```python
from build123d import *

# Parameters (mm, degrees)
F0_R     = 57.15
F0_R_2   = 5
F1_DEPTH = 15
F2_R     = 9.345244
F2_R_2   = 5.10775
F3_DEPTH = 15
F4_R     = 3
F5_DEPTH = 12.7
F6_R     = 1.5
F7_DEPTH = 10


with BuildPart() as f1:
    # F0 (on Front) → F1 (new body)
    with BuildSketch(Plane.XZ):
        Circle(F0_R)
        Circle(F0_R_2, mode=Mode.SUBTRACT)
    extrude(amount=F1_DEPTH)

    # F2 (on face) → F3 (join)
    with BuildSketch(Plane.XZ.offset(15)):
        Circle(F2_R)
        Circle(F2_R_2, mode=Mode.SUBTRACT)
    extrude(amount=F3_DEPTH)

    # F4 (on Top) → F5 (cut, symmetric)
    with BuildSketch(Plane.XY):
        with Locations((0, -23.08)):
            Circle(F4_R)
    extrude(amount=F5_DEPTH, both=True, mode=Mode.SUBTRACT)

    # F6 (on face) → F7 (join)
    with BuildSketch(Plane(origin=(0, 0, 0), x_dir=(-1, 0, 0), z_dir=(0, 1, 0))):
        with Locations((0, 10)):
            Circle(F6_R)
        with Locations((7.071068, 7.071068)):
            Circle(F6_R)
        with Locations((10, 0)):
            Circle(F6_R)
        with Locations((7.071068, -7.071068)):
            Circle(F6_R)
        with Locations((0, -10)):
            Circle(F6_R)
        with Locations((-10, 0)):
            Circle(F6_R)
        with Locations((-7.071068, -7.071068)):
            Circle(F6_R)
        with Locations((-7.071068, 7.071068)):
            Circle(F6_R)
    extrude(amount=F7_DEPTH)


solid = f1.part
```
Source: CAD feature listing. Evaluate the final solid. Frame: model axes, mm. A direction names the side the tool comes from. Round coordinates to 2 decimals unless told otherwise and drop trailing zeros. Loops run counter-clockwise (first coordinate to the right, second up) from the corner with the lowest first, then second, coordinate; pieces in that order, holes last. Notation, with made-up numbers: (-0.5, 33.5) - (40.5, 33.5) arc R19 ccw to (40.5, 44.5) - close; hole circle Ø4 at (-24, 56). An arc over 180 degrees is marked (long way). Use CSV: the item, a comma, the result in double quotes.
Q1. Section query C-C, the plane y = 3. Output: boundary loops of the cut face in (x, z).
Reported:
outline,"circle Ø3 at (-10, 0); circle Ø3 at (-7.07, -7.07); circle Ø3 at (-7.07, 7.07); circle Ø3 at (0, -10); circle Ø3 at (0, 10); circle Ø3 at (7.07, -7.07); circle Ø3 at (7.07, 7.07); circle Ø3 at (10, 0)"
Q2. Section query A-A, the plane z = 0. Output: boundary loops of the cut face in (x, y).
Reported:
outline,"(-57.15, -15) - (-9.35, -15) - (-9.35, -30) - (-5.11, -30) - (-5.11, -15) - (-5, -15) - (-5, 0) - (-8.5, 0) - (-8.5, 10) - (-11.5, 10) - (-11.5, 0) - (-57.15, 0) - close; (5, -15) - (5.11, -15) - (5.11, -30) - (9.35, -30) - (9.35, -15) - (57.15, -15) - (57.15, 0) - (11.5, 0) - (11.5, 10) - (8.5, 10) - (8.5, 0) - (5, 0) - close"
Q3. Section query D-D, the plane y = -7.5. Output: boundary loops of the cut face in (x, z), then the cut area to 3 significant figures.
Reported:
outline,"circle Ø114.3 at (0, 0); hole circle Ø10 at (0, 0)"
area,"10,200 mm^2"
Q4. Section query B-B, the plane x = 0. Give the number of separate pieces and of enclosed holes in the cut face, then the cut area to 3 significant figures.
Reported:
separate pieces,"4"
enclosed holes,"0"
area,"1,700 mm^2"
Q5. Ray query, line 1 along Y through (x, z) = (0, 7); line 2 along X through (y, z) = (-23.08, 7.5); line 3 along Z through (x, y) = (0, -10.75). Return the intervals inside material, ascending.
Reported:
line 1,"-30 to -26.08, -20.08 to 0"
line 2,"-5.58 to -3, 3 to 5.58"
line 3,"-57.15 to -5, 5 to 57.15"
Q6. Mould query, pull axis Z, two halves, no side actions, for faces 1 (the cylindrical face through (4.31, -22.4, -8.29)), 2 (the cylindrical face through (-1.08, -7.4, -4.88)), 3 (the flat face through (-7, 10, 7)). Classes: pulls with the +Z half, pulls with the -Z half, needs draft (parallel to the pull), parting line crosses it, or undercut.
Reported:
face 1,"parting line crosses it"
face 2,"undercut"
face 3,"needs draft"
Q7. Reachability of faces 4 (the cylindrical face through (11.5, 4.93, 0.07)), 5 (the cylindrical face through (2.86, -22.18, 6.78)) from +Z, -Z, +X, -X, +Y, -Y: full face, straight path, thin tool, end or side. Return the list, or none.
Reported:
face 4,"+Y"
face 5,"+Z, -Z"
Q8. Pin query (flat end, axial travel): pin 1 Ø8 at (x, y) = (0, -23.08) entering from +Z; pin 2 Ø1.5 at (x, z) = (-19, 23.5) entering from -Y; pin 3 Ø6 at (y, z) = (-9.5, -29) entering from +X; pin 4 Ø9 at (x, z) = (0, 0) entering from +Y. Return the tip coordinate at first contact, or that it passes through.
Reported:
pin 1,"z = 9.35"
pin 2,"y = -15"
pin 3,"x = 50.89"
pin 4,"through"
